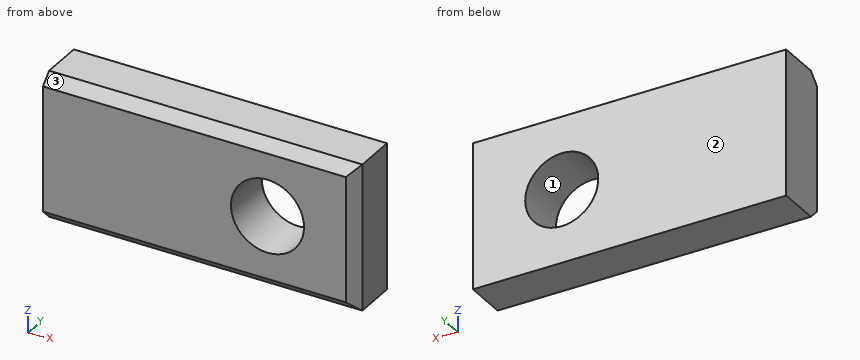
from build123d import *

# Parameters (mm, degrees)
F0_W     = 30
F0_H     = 14
F1_DEPTH = 5
F2_R     = 3.5
F3_DEPTH = 5.001
F4_SIZE  = 1


with BuildPart() as f1:
    # F0 (on Front) → F1 (new body)
    with BuildSketch(Plane.XZ):
        with Locations((15, 7)):
            Rectangle(F0_W, F0_H)
    extrude(amount=F1_DEPTH)

    # F2 (on face) → F3 (cut, through all)
    with BuildSketch(Plane.XZ.offset(5)):
        with Locations((21.5, 7)):
            Circle(F2_R)
    extrude(amount=-F3_DEPTH, mode=Mode.SUBTRACT)

    # F4
    f4_edges = [f1.edges().sort_by_distance(p)[0] for p in [
        (15, -5, 14),
        (30, -5, 7),
        (15, -5, 0),
    ]]
    chamfer(f4_edges, length=F4_SIZE)


solid = f1.part
Geometry check sheet. Reference: the model listing, model coordinates, mm. Face numbers are marked on the shaded views. Round coordinates to 2 decimals unless told otherwise and drop trailing zeros. Order: outer loops, then holes, each group sorted by start corner. A loop starts at its lowest first (then second) coordinate and runs counter-clockwise, first axis right, second up. Notation, with made-up numbers: M 75.5,-10.75 L 91.5,-10.75 A32 cw 91.5,28.25 Z; hole C 72.25,35 d9. An arc over 180 degrees is marked long. Answer in a Markdown table with one row per item.
(1) Scan lines: probe 1 along Z at (x, y) = (21.5, -1.7); probe 2 along X at (y, z) = (-1, 5.25); probe 3 along Z at (x, y) = (22.75, -1.3). Record each from-to range of solid material in increasing order. Write a range as from..to.
Responses:
| item | result |
|---|---|
| probe 1 | z = 0..3.5, 10.5..14 |
| probe 2 | x = 0..18.47, 24.53..30 |
| probe 3 | z = 0..3.73, 10.27..14 |
(2) Sectioned sample at B-B, the plane z = 7. Record the cut outline in (x, y).
Responses:
| item | result |
|---|---|
| outline | M 0,-5 L 18,-5 L 18,0 L 0,0 Z; M 25,-5 L 29,-5 L 30,-4 L 30,0 L 25,0 Z |
(3) Draft check along Z on the marked faces 1, 2 and 3. Enter one of: released by +Z, released by -Z, zero draft, split by the parting line, or undercut.
Responses:
| item | result |
|---|---|
| face 1 | undercut |
| face 2 | zero draft |
| face 3 | released by +Z |
(4) Sectioned sample at C-C, the plane y = -1.1. Record the cut outline in (x, z).
Responses:
| item | result |
|---|---|
| outline | M 0,0 L 30,0 L 30,14 L 0,14 Z; hole C 21.5,7 d7 |
(5) Sectioned sample at A-A, the plane x = 21.5. Record the cut outline in (y, z).
Responses:
| item | result |
|---|---|
| outline | M -5,1 L -4,0 L 0,0 L 0,3.5 L -5,3.5 Z; M -5,10.5 L 0,10.5 L 0,14 L -4,14 L -5,13 Z |
